Here's how the part is built. I have some questions about the finished solid (model axes, mm). Coordinates: 2 decimals unless noted, no trailing zeros. Write each loop counter-clockwise with the first axis right and the second up, starting at its lowest first coordinate (ties: lowest second). Pieces come first, ordered by that corner, then holes.
Item 1: If I drill on line 1 (Z direction, x = -83, y = 5.75), over which ranges is the centre line in solid material (lowest first)?
Item 2: I'm going to push flat-ended pins straight in: pin 1 Ø1.9 at (x, y) = (-226.5, 4.5) entering from +Z; pin 2 Ø3 at (y, z) = (4.5, 74) entering from +X; pin 3 Ø1.9 at (y, z) = (2, -71.5) entering from -X. Where does each tip first touch, or does it pass through?
Item 3: If we section it at A-A (x = -255): Please give me the cut outline in (y, z).
from build123d import *

# Parameters (mm, degrees)
SKETCH1_W                 = 721.63658441
SKETCH1_H                 = 152.4
BOSS_EXTRUDE1_DEPTH       = 6.35
SKETCH2_W                 = 39.679316882
SKETCH2_H                 = 6.35
SKETCH2_W_2               = 31.750000127
CUT_EXTRUDE1_DEPTH        = 7.35
LPATTERN1_COUNT           = 3
LPATTERN1_PITCH           = 153.979316882
LPATTERN1_COL_COUNT       = 3
LPATTERN1_COL_PITCH       = 153.979316882
MIRROR1_COPY_1_SKETCH_W   = 39.679316882
MIRROR1_COPY_1_SKETCH_H   = 6.35
MIRROR1_COPY_1_SKETCH_W_2 = 31.750000127
MIRROR1_COPY_1_DEPTH      = 7.35
MIRROR1_COPY_2_SKETCH_W   = 39.679316882
MIRROR1_COPY_2_SKETCH_H   = 6.35
MIRROR1_COPY_2_SKETCH_W_2 = 31.750000127
MIRROR1_COPY_2_DEPTH      = 7.35
MIRROR1_COPY_3_SKETCH_W   = 39.679316882
MIRROR1_COPY_3_SKETCH_H   = 6.35
MIRROR1_COPY_3_SKETCH_W_2 = 31.750000127
MIRROR1_COPY_3_DEPTH      = 7.35
MIRROR1_COPY_4_SKETCH_W   = 39.679316882
MIRROR1_COPY_4_SKETCH_H   = 6.35
MIRROR1_COPY_4_SKETCH_W_2 = 31.750000127
MIRROR1_COPY_4_DEPTH      = 7.35
CUT_EXTRUDE2_DEPTH        = 7.35


with BuildPart() as part:
    # Sketch1 → Boss-Extrude1 (new body)
    with BuildSketch(Plane(origin=(0, 0, 0), x_dir=(1, 0, 0), z_dir=(0, 1, 0))):
        Rectangle(SKETCH1_W, SKETCH1_H)
    extrude(amount=BOSS_EXTRUDE1_DEPTH)

    # Sketch2 → Cut-Extrude1 (cut, through all)
    with BuildSketch(Plane(origin=(0, 6.35, 0), x_dir=(1, 0, 0), z_dir=(0, 1, 0))):
        with Locations((0, -73.025)):
            Rectangle(SKETCH2_W, SKETCH2_H)
        with Locations((-61.114658505, -73.025)):
            Rectangle(SKETCH2_W_2, SKETCH2_H)
        with Locations((61.114658505, -73.025)):
            Rectangle(SKETCH2_W_2, SKETCH2_H)
    cut_extrude1 = extrude(amount=-CUT_EXTRUDE1_DEPTH, mode=Mode.SUBTRACT)

    # LPattern1: Cut-Extrude1 ×3
    with Locations(*[(i * LPATTERN1_PITCH, 0, 0) for i in range(1, LPATTERN1_COUNT)]):
        add(cut_extrude1, mode=Mode.SUBTRACT)

    # LPattern1 col: Cut-Extrude1 ×3
    with Locations(*[(-i * LPATTERN1_COL_PITCH, 0, 0) for i in range(1, LPATTERN1_COL_COUNT)]):
        add(cut_extrude1, mode=Mode.SUBTRACT)

    # Mirror1: Cut-Extrude1 across plane
    add(cut_extrude1.mirror(Plane.XY), mode=Mode.SUBTRACT)

    # Mirror1 copy 1 sketch → Mirror1 copy 1 (cut, through all)
    with BuildSketch(Plane(origin=(153.979316882, 6.35, 0), x_dir=(1, 0, 0), z_dir=(0, 1, 0))):
        with Locations((0, 73.025)):
            Rectangle(MIRROR1_COPY_1_SKETCH_W, MIRROR1_COPY_1_SKETCH_H)
        with Locations((-61.114658505, 73.025)):
            Rectangle(MIRROR1_COPY_1_SKETCH_W_2, MIRROR1_COPY_1_SKETCH_H)
        with Locations((61.114658505, 73.025)):
            Rectangle(MIRROR1_COPY_1_SKETCH_W_2, MIRROR1_COPY_1_SKETCH_H)
    extrude(amount=-MIRROR1_COPY_1_DEPTH, mode=Mode.SUBTRACT)

    # Mirror1 copy 2 sketch → Mirror1 copy 2 (cut, through all)
    with BuildSketch(Plane(origin=(307.958633764, 6.35, 0), x_dir=(1, 0, 0), z_dir=(0, 1, 0))):
        with Locations((0, 73.025)):
            Rectangle(MIRROR1_COPY_2_SKETCH_W, MIRROR1_COPY_2_SKETCH_H)
        with Locations((-61.114658505, 73.025)):
            Rectangle(MIRROR1_COPY_2_SKETCH_W_2, MIRROR1_COPY_2_SKETCH_H)
        with Locations((61.114658505, 73.025)):
            Rectangle(MIRROR1_COPY_2_SKETCH_W_2, MIRROR1_COPY_2_SKETCH_H)
    extrude(amount=-MIRROR1_COPY_2_DEPTH, mode=Mode.SUBTRACT)

    # Mirror1 copy 3 sketch → Mirror1 copy 3 (cut, through all)
    with BuildSketch(Plane(origin=(-153.979316882, 6.35, 0), x_dir=(1, 0, 0), z_dir=(0, 1, 0))):
        with Locations((0, 73.025)):
            Rectangle(MIRROR1_COPY_3_SKETCH_W, MIRROR1_COPY_3_SKETCH_H)
        with Locations((-61.114658505, 73.025)):
            Rectangle(MIRROR1_COPY_3_SKETCH_W_2, MIRROR1_COPY_3_SKETCH_H)
        with Locations((61.114658505, 73.025)):
            Rectangle(MIRROR1_COPY_3_SKETCH_W_2, MIRROR1_COPY_3_SKETCH_H)
    extrude(amount=-MIRROR1_COPY_3_DEPTH, mode=Mode.SUBTRACT)

    # Mirror1 copy 4 sketch → Mirror1 copy 4 (cut, through all)
    with BuildSketch(Plane(origin=(-307.958633764, 6.35, 0), x_dir=(1, 0, 0), z_dir=(0, 1, 0))):
        with Locations((0, 73.025)):
            Rectangle(MIRROR1_COPY_4_SKETCH_W, MIRROR1_COPY_4_SKETCH_H)
        with Locations((-61.114658505, 73.025)):
            Rectangle(MIRROR1_COPY_4_SKETCH_W_2, MIRROR1_COPY_4_SKETCH_H)
        with Locations((61.114658505, 73.025)):
            Rectangle(MIRROR1_COPY_4_SKETCH_W_2, MIRROR1_COPY_4_SKETCH_H)
    extrude(amount=-MIRROR1_COPY_4_DEPTH, mode=Mode.SUBTRACT)

    # Sketch3 → Cut-Extrude2 (cut, through all)
    with BuildSketch(Plane(origin=(0, 6.35, 0), x_dir=(1, 0, 0), z_dir=(0, 1, 0))):
        Polygon((307.958633764, 69.85), (307.958633764, -76.2), (360.818292205, -76.2), (360.818292205, 76.2), (307.958633764, 76.2), align=None)
    extrude(amount=-CUT_EXTRUDE2_DEPTH, mode=Mode.SUBTRACT)


solid = part.part
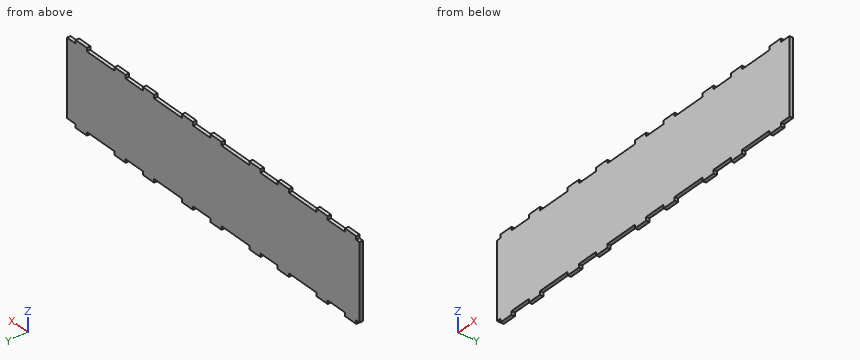
Answer list:
1. line 1: z = -69.85 to 69.85
2. pin 1: stops at z = 69.85
2. pin 2: stops at x = 288.12
2. pin 3: stops at x = -353.2
3. outline: (0, -69.85) - (6.35, -69.85) - (6.35, 69.85) - (0, 69.85) - close
